```python
from build123d import *

# Parameters (mm, degrees)
RESSALTO_EXTRUS_O1_DEPTH = 20
CORTE_EXTRUS_O1_DEPTH    = 6
ESBO_O3_R                = 3.25
CORTE_EXTRUS_O2_DEPTH    = 18.170032033


with BuildPart() as part:
    # Esboço1 → Ressalto-extrusão1 (new body)
    with BuildSketch(Plane(origin=(0, 0, 0), x_dir=(1, 0, 0), z_dir=(0, 1, 0))):
        Polygon((-8, 2.5), (-6.156497116, 2.5), (-2.756497116, 5.9), (2.756497116, 5.9), (6.156497116, 2.5), (8, 2.5), (8, -2.5), (6.156497116, -2.5), (2.756497116, -5.9), (-2.756497116, -5.9), (-6.156497116, -2.5), (-8, -2.5), align=None)
    extrude(amount=RESSALTO_EXTRUS_O1_DEPTH)

    # Esboço2 → Corte-extrusão1 (cut)
    with BuildSketch(Plane(origin=(0, 20, 0), x_dir=(1, 0, 0), z_dir=(0, 1, 0))):
        Polygon((-3.290896534, 5.7), (-3.290896534, 6.558868729), (3.290896534, 6.558868729), (3.290896534, 5.7), (6.581793069, 0), (3.290896534, -5.7), (3.290896534, -6.558868729), (-3.290896534, -6.558868729), (-3.290896534, -5.7), (-6.581793069, 0), align=None)
    extrude(amount=-CORTE_EXTRUS_O1_DEPTH, mode=Mode.SUBTRACT)

    # Esboço3 → Corte-extrusão2 (cut, through all)
    with BuildSketch(Plane(origin=(0, 14, 0), x_dir=(1, 0, 0), z_dir=(0, 1, 0))):
        with Locations(Location((0, 0, 0), (0, 0, 270))):
            Circle(ESBO_O3_R)
    extrude(amount=-CORTE_EXTRUS_O2_DEPTH, mode=Mode.SUBTRACT)


solid = part.part
```
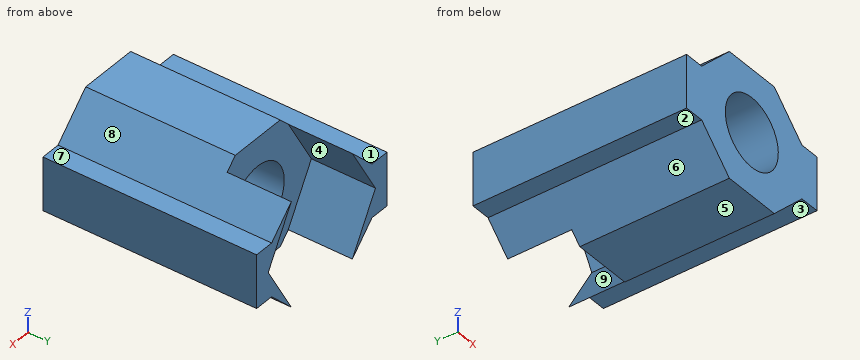
Design review of the part built by this model. Coordinates are the model's own, in mm. Face numbers are marked on the shaded views. A direction names the side the tool comes from. Give positions to 0.01 mm unless a question says otherwise; leave off trailing zeros. Order: outer loops, then holes, each group sorted by start corner. A loop starts at its lowest first (then second) coordinate and runs counter-clockwise, first axis right, second up. Notation, with made-up numbers: (-37.5, 77) -> (7.5, 77) arc R14 cw to (7.5, 99) -> close; hole circle Ø7 at (72, 65). An arc over 180 degrees is marked (long way). Write item = value, one per line. Start each with the question number.
(1) We need section D-D on z = 2. Write out the cut boundary in (x, y), plus the area to 3 significant figures.
(2) We need section B-B on x = 0. Write out the cut boundary in (y, z), plus the area to 3 significant figures.
(3) To check wall thickness, follow line 1 along X through (y, z) = (5.5, 0); line 2 along X through (y, z) = (15.5, -4); line 3 along Z through (x, y) = (-6.75, 11.75). State the ranges of each line that lie inside material, in increasing order.
(4) Mouldability with a two-part tool opening along X and no side actions: class the marked faces 6, 7, 8 and 9 as +X half, -X half, draft (parallel to the pull), parting line (faces both ways), or undercut.
(5) For the marked faces 1, 2, 3, 4 and 5, list the 3-axis set-ups (+Z, -Z, +X, -X, +Y, -Y) from which the entire face can be reached by the end or side of a thin tool; tool diameter is ignored.
(6) For pin 1 (0.9 mm diameter, centred on x = 7, y = 12.5, fed in from +Z); pin 2 (2 mm diameter, centred on x = -7, y = 6, fed in from -Z); pin 3 (0.9 mm diameter, centred on x = -6.5, y = 9.5, fed in from +Z), all flat-tipped, find the tip position at first contact; note any pin that passes through.
(7) We need section C-C on y = 7.25. Write out the cut boundary in (x, z).
(8) We need section A-A on y = 14.5. Write out the cut boundary in (x, z), plus the area to 3 significant figures.
Numbers:
q1.outline = (-8, 0) -> (-2.56, 0) -> (-2.56, 14) -> (-5.43, 14) -> (-5.43, 20) -> (-8, 20) -> close; (2.56, 0) -> (8, 0) -> (8, 20) -> (5.43, 20) -> (5.43, 14) -> (2.56, 14) -> close
q1.area = 183 mm^2
q2.outline = (0, -5.9) -> (14, -5.9) -> (14, -3.25) -> (0, -3.25) -> close; (0, 3.25) -> (14, 3.25) -> (14, 5.9) -> (0, 5.9) -> close
q2.area = 74.2 mm^2
q3.line_1 = -8 to -3.25, 3.25 to 8
q3.line_2 = -4.66 to -4.27, 4.27 to 4.66
q3.line_3 = -2.5 to 2.5
q4.face_6 = -X half
q4.face_7 = draft
q4.face_8 = +X half
q4.face_9 = undercut
q5.face_1 = +Z, -X, +Y, -Y
q5.face_2 = -Z, -X, +Y, -Y
q5.face_3 = -Z, +X, +Y, -Y
q5.face_4 = +Y
q5.face_5 = -Z, +X, -X, +Y, -Y
q6.pin_1 = 2.5
q6.pin_2 = -2.66
q6.pin_3 = 2.61
q7.outline = (-8, -2.5) -> (-6.16, -2.5) -> (-2.76, -5.9) -> (2.76, -5.9) -> (6.16, -2.5) -> (8, -2.5) -> (8, 2.5) -> (6.16, 2.5) -> (2.76, 5.9) -> (-2.76, 5.9) -> (-6.16, 2.5) -> (-8, 2.5) -> close; hole circle Ø6.5 at (0, 0)
q8.outline = (-8, -2.5) -> (-6.16, -2.5) -> (-3.75, -4.91) -> (-6.58, 0) -> (-3.75, 4.91) -> (-6.16, 2.5) -> (-8, 2.5) -> close; (3.75, -4.91) -> (6.16, -2.5) -> (8, -2.5) -> (8, 2.5) -> (6.16, 2.5) -> (3.75, 4.91) -> (6.58, 0) -> close
q8.area = 26.3 mm^2
